```python
from build123d import *

# Parameters (mm, degrees)
EXTRUDE_1_DEPTH     = 20
SKETCH_2_R          = 13
CUT_EXTRUDE_1_DEPTH = 12
SKETCH_3_R          = 4
CUT_EXTRUDE_2_DEPTH = 49.808298475


with BuildPart() as part:
    # 草图1 → 凸台-拉伸1 (new, symmetric)
    with BuildSketch(Plane.XY):
        with BuildLine():
            Line((-5, 0), (5, 0))
            Line((5, 0), (5, 4))
            Line((5, 4), (20, 4))
            Line((20, 4), (20, 0))
            Line((20, 0), (37.5, 0))
            Line((37.5, 0), (37.5, 10))
            Line((37.5, 10), (25, 10))
            Line((25, 10), (25, 34))
            Line((25, 34), (20, 34))
            Line((20, 34), (20, 30))
            Line((20, 30), (10, 30))
            ThreePointArc((10, 30), (0, 20), (-10, 30))
            Line((-10, 30), (-20, 30))
            Line((-20, 30), (-20, 34))
            Line((-20, 34), (-25, 34))
            Line((-25, 34), (-25, 10))
            Line((-25, 10), (-37.5, 10))
            Line((-37.5, 10), (-37.5, 0))
            Line((-37.5, 0), (-20, 0))
            Line((-20, 0), (-20, 4))
            Line((-20, 4), (-5, 4))
            Line((-5, 4), (-5, 0))
        make_face()
    extrude(amount=EXTRUDE_1_DEPTH, both=True)

    # 草图2 → 切除-拉伸1 (cut, symmetric)
    with BuildSketch(Plane.XY):
        with Locations((0, 30)):
            Circle(SKETCH_2_R)
    extrude(amount=CUT_EXTRUDE_1_DEPTH, both=True, mode=Mode.SUBTRACT)

    # 草图3 → 切除-拉伸2 (cut, through all)
    with BuildSketch(Plane(origin=(0, 10, 0), x_dir=(1, 0, 0), z_dir=(0, 1, 0))):
        with Locations(Location((-32.5, 0, 0), (0, 0, 180))):
            Circle(SKETCH_3_R)
        with Locations(Location((32.5, 0, 0), (0, 0, 180))):
            Circle(SKETCH_3_R)
    extrude(amount=-CUT_EXTRUDE_2_DEPTH, mode=Mode.SUBTRACT)


solid = part.part
```
Read the model definition and answer for the solid it produces. Units are mm, in the model's axes. A direction names the side the tool comes from. Round coordinates to 2 decimals unless told otherwise and drop trailing zeros. Write each loop counter-clockwise with the first axis right and the second up, starting at its lowest first coordinate (ties: lowest second). Pieces come first, ordered by that corner, then holes. Notation, with made-up numbers: (22.25, 41) -> (49.25, 41) arc R23 ccw to (49.25, 70) -> close; hole circle Ø9 at (-24.5, 22.25). An arc over 180 degrees is marked (long way). Answer in a Markdown table with one row per item. Add a question column.
1) Determine the mould class of faces 1 (the face through (-1, 13, 20)), 2 (the face through (-0.1, 19.7, -12)), 3 (the face through (-37.5, 5, 0)), 4 (the face through (25, 22, 0)) for opening direction X: pulls with the +X half, pulls with the -X half, needs draft (parallel to the pull), parting line crosses it, or undercut.
2) Which of the six approach directions +Z, -Z, +X, -X, +Y, -Y give full straight-line access (tool end or side, diameter ignored) to faces 5 (the face through (-25, 22, 0)), 6 (the face through (-20, 2, 0)), 7 (the face through (20, 32, 0))?
3) Find section D-D, the plane y = 12. Determine the outline of the cut face in (x, z).
4) Given P1, Ø4, axis at x = -2.5, y = 21.5, coming from the -Z side; P2, Ø12, axis at y = 23.5, z = 11, coming from the +X side; P3, Ø4, axis at x = -29, z = 9, coming from the +Y side; P4, Ø6, axis at y = 15.5, z = 14, coming from the -X side, each flat-ended and moving along its own axis, determine where each tip first touches the part or whether it passes through.
5) Find section B-B, the plane x = 32.5. Determine the outline of the cut face in (y, z).
6) Find section A-A, the plane z = 0. State how many separate pieces and enclosed holes the cut face has, and give its area (3 significant figures).
7) Consider line 1 (X direction, y = 2.5, z = -15); line 2 (Z direction, x = 32.5, y = 7.5); line 3 (Y direction, x = 19, z = 11). Determine where each line is inside the solid, lowest interval first.
8) Find section C-C, the plane z = -8. Determine the outline of the cut face in (x, y), and give its area (3 significant figures).
Findings below:
| question | item | result |
|---|---|---|
| 1 | face 1 | needs draft |
| 1 | face 2 | undercut |
| 1 | face 3 | pulls with the -X half |
| 1 | face 4 | pulls with the +X half |
| 2 | face 5 | +Z, -Z, -X, +Y |
| 2 | face 6 | +Z, -Z, -Y |
| 2 | face 7 | +Z, -Z, +Y |
| 3 | outline | (-25, -20) -> (25, -20) -> (25, 20) -> (-25, 20) -> close |
| 4 | P1 | z = -20 |
| 4 | P2 | x = 25 |
| 4 | P3 | y = 10 |
| 4 | P4 | x = -25 |
| 5 | outline | (0, -20) -> (10, -20) -> (10, -4) -> (0, -4) -> close; (0, 4) -> (10, 4) -> (10, 20) -> (0, 20) -> close |
| 6 | separate pieces | 3 |
| 6 | enclosed holes | 0 |
| 6 | area | 1,240 mm² |
| 7 | line 1 | -37.5 to -20, -5 to 5, 20 to 37.5 |
| 7 | line 2 | -20 to -4, 4 to 20 |
| 7 | line 3 | 4 to 30 |
| 8 | outline | (-37.5, 0) -> (-20, 0) -> (-20, 4) -> (-5, 4) -> (-5, 0) -> (5, 0) -> (5, 4) -> (20, 4) -> (20, 0) -> (37.5, 0) -> (37.5, 10) -> (25, 10) -> (25, 34) -> (20, 34) -> (20, 30) -> (13, 30) arc R13 cw to (-13, 30) -> (-20, 30) -> (-20, 34) -> (-25, 34) -> (-25, 10) -> (-37.5, 10) -> close |
| 8 | area | 1,400 mm² |
